Work out the finished part from the listing and answer in its coordinate system (mm). A direction names the side the tool comes from. Round coordinates to 2 decimals unless told otherwise and drop trailing zeros. Loops run counter-clockwise (first coordinate to the right, second up) from the corner with the lowest first, then second, coordinate; pieces in that order, holes last. Notation, with made-up numbers: (-38, -31) -> (1, -31) arc R29 cw to (1, 3) -> close; hole circle Ø7 at (-17, -17.75). An arc over 180 degrees is marked (long way). Use one line per item in the form item = value.
```python
from build123d import *

# Parameters (mm, degrees)
SKETCH_9_R                  = 1.5
EXTRUDE_4_DEPTH             = 15
EXTRUDE_4_DEPTH_BACK        = 15
EXTRUDE_5_REACH             = 17
SKETCH_10_R                 = 1.5
EXTRUDE_5_DIRECTION_2_REACH = 17
HOLE_WIZARD_M52_AT_2_COUNT  = 2
HOLE_WIZARD_M52_AT_2_PITCH  = 14
HOLE_WIZARD_M51_D           = 5.5
HOLE_WIZARD_M51_CSINK_D     = 10.4
HOLE_WIZARD_M51_CSINK_ANGLE = 90
CUT_EXTRUDE_3_DEPTH         = 16
CUT_EXTRUDE_3_DEPTH_BACK    = 16
SKETCH_25_W                 = 0.5
SKETCH_25_H                 = 7.5
CUT_EXTRUDE_7_DEPTH         = 13.794228634
SKETCH_27_W                 = 0.5
SKETCH_27_H                 = 7.5
CUT_EXTRUDE_8_DEPTH         = 5
FILLET_4_R                  = 3


with BuildPart() as part:
    # Sketch 9 → Extrude 4 (new body, two sides)
    with BuildSketch(Plane(origin=(0, 0, 0), x_dir=(1, 0, 0), z_dir=(0, 1, 0))) as extrude_4_sk:
        with BuildLine():
            Line((0, 4), (18, 4))
            Line((18, 4), (18, 0))
            Line((18, 0), (4, 0))
            ThreePointArc((4, 0), (-2.828427125, -2.828427125), (0, 4))
        make_face()
        with Locations(Location((0, 0, 0), (0, 0, 270))):  # turned: the seam where the file's is
            Circle(SKETCH_9_R, mode=Mode.SUBTRACT)
    extrude(amount=EXTRUDE_4_DEPTH)
    extrude(extrude_4_sk.sketch, amount=-EXTRUDE_4_DEPTH_BACK)

    # Extrude 5: up to this face of the body (flat: up to its plane)
    extrude_5_end = Plane(part.part.faces().sort_by_distance((6.10604541, 15, -1.19522591))[0])
    # Sketch 10 → Extrude 5 (add, up to the picked face)
    with BuildSketch(Plane(origin=(0, 0, 0), x_dir=(1, 0, 0), z_dir=(0, 1, 0)), mode=Mode.PRIVATE) as extrude_5_sk1:
        with BuildLine():
            Line((-3.464101615, 2), (-12.464101615, -13.588457268))
            Line((-12.464101615, -13.588457268), (-9, -15.588457268))
            Line((-9, -15.588457268), (-2, -3.464101615))
            ThreePointArc((-2, -3.464101615), (3.863703305, 1.03527618), (-3.464101615, 2))
        make_face()
        with Locations(Location((0, 0, 0), (0, 0, 270))):  # turned: the seam where the file's is
            Circle(SKETCH_10_R, mode=Mode.SUBTRACT)
    extrude_5_tool1 = split(extrude(extrude_5_sk1.sketch, amount=EXTRUDE_5_REACH, mode=Mode.PRIVATE), bisect_by=extrude_5_end, keep=Keep.BOTH, mode=Mode.PRIVATE)
    add(extrude_5_tool1.solids().sort_by(Axis((-4.088119, 0, 4.690377), (0, 1, 0)))[0])

    # Extrude 5 direction 2: up to this face of the body (flat: up to its plane)
    extrude_5_direction_2_end = Plane(part.part.faces().sort_by_distance((6.10604541, -15, -1.19522591))[0])
    # Sketch 10 → Extrude 5 direction 2 (add, up to the picked face)
    with BuildSketch(Plane(origin=(0, 0, 0), x_dir=(1, 0, 0), z_dir=(0, 1, 0)), mode=Mode.PRIVATE) as extrude_5_direction_2_sk1:
        with BuildLine():
            Line((-3.464101615, 2), (-12.464101615, -13.588457268))
            Line((-12.464101615, -13.588457268), (-9, -15.588457268))
            Line((-9, -15.588457268), (-2, -3.464101615))
            ThreePointArc((-2, -3.464101615), (3.863703305, 1.03527618), (-3.464101615, 2))
        make_face()
        with Locations(Location((0, 0, 0), (0, 0, 270))):  # turned: the seam where the file's is
            Circle(SKETCH_10_R, mode=Mode.SUBTRACT)
    extrude_5_direction_2_tool1 = split(extrude(extrude_5_direction_2_sk1.sketch, amount=-EXTRUDE_5_DIRECTION_2_REACH, mode=Mode.PRIVATE), bisect_by=extrude_5_direction_2_end, keep=Keep.BOTH, mode=Mode.PRIVATE)
    add(extrude_5_direction_2_tool1.solids().sort_by(Axis((-4.088119, 0, 4.690377), (0, -1, 0)))[0])

    # Sketch 12 → Hole Wizard M52 (revolve, cut)
    with BuildSketch(Plane(origin=(10, 7, 0), x_dir=(0, -1, 0), z_dir=(1, 0, 0))):
        Polygon((0, 0), (0, 4), (2.75, 4), (2.75, 2.45), (5.2, 0), align=None)
    hole_wizard_m52 = revolve(axis=Axis((10, 7, 6.35), (0, 0, -1)), mode=Mode.SUBTRACT)

    # Hole Wizard M52 at 2: Hole Wizard M52 ×2
    with Locations(*[(0, -i * HOLE_WIZARD_M52_AT_2_PITCH, 0) for i in range(1, HOLE_WIZARD_M52_AT_2_COUNT)]):
        add(hole_wizard_m52, mode=Mode.SUBTRACT)

    # Hole Wizard M51 (through all)
    with Locations(Plane(origin=(0, 0, 0), x_dir=(0.5, 0, -0.866025404), z_dir=(0.866025404, 0, 0.5))):
        with Locations((-10, 7), (-10, -7)):
            CounterSinkHole(HOLE_WIZARD_M51_D / 2, HOLE_WIZARD_M51_CSINK_D / 2, counter_sink_angle=HOLE_WIZARD_M51_CSINK_ANGLE)

    # Sketch 17 → Cut-Extrude 3 (cut, two sides)
    with BuildSketch(Plane(origin=(0, 0, 0), x_dir=(1, 0, 0), z_dir=(0, 1, 0))) as cut_extrude_3_sk:
        with BuildLine():
            Line((-2, -3.464101615), (-1.75, -3.031088913))
            ThreePointArc((-1.75, -3.031088913), (1.75, -3.031088913), (3.5, 0))
            Line((3.5, 0), (4, 0))
            ThreePointArc((4, 0), (2, -3.464101615), (-2, -3.464101615))
        make_face()
    extrude(amount=CUT_EXTRUDE_3_DEPTH, mode=Mode.SUBTRACT)
    extrude(cut_extrude_3_sk.sketch, amount=-CUT_EXTRUDE_3_DEPTH_BACK, mode=Mode.SUBTRACT)

    # Sketch 25 → Cut-Extrude 7 (cut, through all)
    with BuildSketch(Plane(origin=(0, 0, 0), x_dir=(0.5, 0, -0.866025404), z_dir=(0.866025404, 0, 0.5))):
        with Locations((-3.75, 11.25)):
            Rectangle(SKETCH_25_W, SKETCH_25_H)
        with Locations((-3.75, -3.75)):
            Rectangle(SKETCH_25_W, SKETCH_25_H)
    extrude(amount=-CUT_EXTRUDE_7_DEPTH, mode=Mode.SUBTRACT)

    # Sketch 27 → Cut-Extrude 8 (cut, through all)
    with BuildSketch(Plane.XY):
        with Locations((3.75, 3.75)):
            Rectangle(SKETCH_27_W, SKETCH_27_H)
        with Locations((3.75, -11.25)):
            Rectangle(SKETCH_27_W, SKETCH_27_H)
    extrude(amount=-CUT_EXTRUDE_8_DEPTH, mode=Mode.SUBTRACT)

    # Fillet 4
    fillet_4_edges = [part.edges().sort_by_distance(p)[0] for p in [
        (18, -15, -2),
        (18, 15, -2),
        (-10.732050808, 15, 14.588457268),
        (-10.732050808, -15, 14.588457268),
    ]]
    fillet(fillet_4_edges, radius=FILLET_4_R)


solid = part.part
```
(1) Given P1, Ø6, axis at y = -3, z = 8, coming from the +X side; P2, Ø11.5, axis at x = 12, y = -3.5, coming from the +Z side; P3, Ø6, axis at y = 10, z = 8.5, coming from the -X side, each flat-ended and moving along its own axis, determine where each tip first touches the part or whether it passes through.
Completed:
P1 = -2.89
P2 = 0
P3 = -11.26
(2) Find section D-D, the plane z = 2. Write down the section's boundary in (x, y).
Completed:
outline = (-5.77, -15) -> (2.87, -15) -> (2.87, 15) -> (-3.54, 15) -> (-3.54, 7.5) -> (-4.54, 7.5) -> (-4.54, 15) -> (-5.77, 15) -> close; hole (-4.54, -7.5) -> (-3.54, -7.5) -> (-3.54, 0) -> (-4.54, 0) -> close
(3) For a pull along Y with two mould halves and no side action, classify faces 4 (the cylindrical face through (9.17, 4.38, -3.21)), 5 (the flat face through (-4, -15, 3)), 6 (the flat face through (11, 0, 0)) as +Y half, -Y half, draft (parallel to the pull), parting line (faces both ways), or undercut.
Completed:
face_4 = undercut
face_5 = -Y half
face_6 = draft
(4) Find section B-B, the plane y = 7. Write down the section's boundary in (x, z), then the cut area to 3 significant figures.
Completed:
outline = (-12.46, 13.59) -> (-9.84, 9.04) -> (-8.5, 9.82) -> (-7.6, 13.16) -> (-9, 15.59) -> close; (-7.09, 4.28) -> (-3.46, -2) arc R4 ccw to (0, -4) -> (3.5, -4) -> (3.5, 0) arc R3.5 ccw to (-1.75, 3.03) -> (-2.4, 4.16) -> (-5.75, 5.05) -> close; (4, -4) -> (7.25, -4) -> (7.25, -2.45) -> (4.8, 0) -> (4, 0) -> close; (12.75, -4) -> (18, -4) -> (18, 0) -> (15.2, 0) -> (12.75, -2.45) -> close; hole circle Ø3 at (0, 0)
area = 100 mm2
(5) Find section A-A, the plane y = -1. Write down the section's boundary in (x, z).
Completed:
outline = (-12.46, 13.59) -> (-5.46, 1.46) -> (-2, 3.46) -> (-9, 15.59) -> close; (-5.21, 1.03) -> (-3.46, -2) arc R4 ccw to (0, -4) -> (18, -4) -> (18, 0) -> (3.5, 0) arc R3.5 ccw to (-1.75, 3.03) -> close; hole circle Ø3 at (0, 0)
(6) Find section C-C, the plane z = -1. Write down the section's boundary in (x, y), then the cut area to 3 significant figures.
Completed:
outline = (-4.04, -15) -> (-1.12, -15) -> (-1.12, 15) -> (-4.04, 15) -> close; (1.12, -15) -> (3.5, -15) -> (3.5, -7.5) -> (4, -7.5) -> (4, -15) -> (15, -15) arc R3 ccw to (18, -12) -> (18, 12) arc R3 ccw to (15, 15) -> (1.12, 15) -> close; hole (3.5, 0) -> (4, 0) -> (4, 7.5) -> (3.5, 7.5) -> close; hole circle Ø8.4 at (10, -7); hole circle Ø8.4 at (10, 7)
area = 472 mm2
(7) For faces 1 (the flat face through (4, -11, -2)), 2 (the cylindrical face through (-10.257, 14.145, 13.821)), 3 (the flat face through (-3.458, -3.802, 2.045)), determine the directions among +Z, -Z, +X, -X, +Y, -Y from which every point of the face is accessible in a straight line to the end or side of a thin tool.
Completed:
face_1 = +Z, -Z, -Y
face_2 = +Z, -X, +Y
face_3 = none
(8) Consider L1, parallel to Y at x = 10, z = -2.8; L2, parallel to X at y = 7, z = -2.9 (3 decimals); L3, parallel to Y at x = -8, z = 10.25. Determine where each line is inside the solid, lowest interval first.
Completed:
L1 = -15 to -9.75, -4.25 to 4.25, 9.75 to 15
L2 = -2.755 to 3.5, 4 to 7.25, 12.75 to 18
L3 = -15 to -8.81, -5.19 to 5.19, 8.81 to 15
